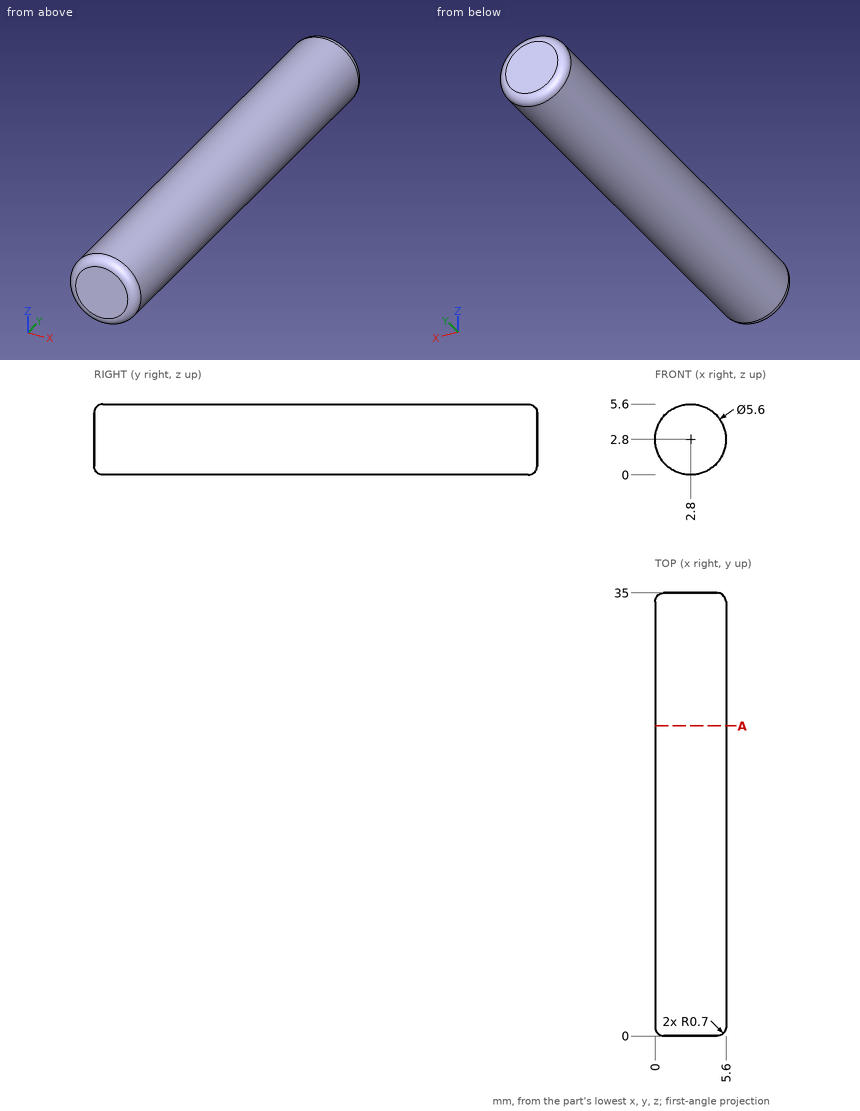
Source: three-view drawing plus pictorial views. Frame: mm from the lowest corner of the part. Give positions to 0.01 mm unless a question says otherwise; leave off trailing zeros. Order: outer loops, then holes, each group sorted by start corner. A loop starts at its lowest first (then second) coordinate and runs counter-clockwise, first axis right, second up. Notation, with made-up numbers: M 15.5,-14 L 54.5,-14 A18 cw 54.5,9 Z; hole C 29,4.25 d4. An arc over 180 degrees is marked long. One line per question, with ' | ' between items. Start each with the question number.
1. Material intervals for probe 1 along X at (y, z) = (10, 2.95); probe 2 along Z at (x, y) = (1, 32); probe 3 along Z at (x, y) = (0.5, 24), sorted ascending. Write a range as [from, to].
2. Section query A-A (y = 24.5). Return the cut outline in (x, z).
3. First-contact query: pin 1 Ø2 at (x, y) = (1.5, 30) entering from -Z; pin 2 Ø3 at (x, y) = (5, 19) entering from +Z; pin 3 Ø3 at (y, z) = (23.5, 5) entering from -X. Flat tips, straight axial feed; report the tip coordinate or a pass-through.
Here are the results:
1) probe 1: [0, 5.6] | probe 2: [0.66, 4.94] | probe 3: [1.2, 4.4]
2) outline: C 2.8,2.8 d5.6
3) pin 1: z = 0.02 | pin 2: z = 5.51 | pin 3: x = 0.09
